Source: CAD feature listing. Evaluate the final solid. Frame: model axes, mm. Coordinates: 2 decimals unless noted, no trailing zeros. One line per question, with ' | ' between items. Start each with the question number.
```python
from build123d import *

# Parameters (mm, degrees)
SKETCH1_W           = 183.7944
SKETCH1_H           = 285.3944
BOSS_EXTRUDE1_DEPTH = 2.9972
SKETCH2_R           = 1.5
BOSS_EXTRUDE2_DEPTH = 2.9972


with BuildPart() as part:
    # Sketch1 → Boss-Extrude1 (new body)
    with BuildSketch(Plane(origin=(0, 0, 0), x_dir=(1, 0, 0), z_dir=(0, 1, 0))):
        Rectangle(SKETCH1_W, SKETCH1_H)
    extrude(amount=BOSS_EXTRUDE1_DEPTH)

    # Sketch2 → Boss-Extrude2 (add)
    # profile 1 of 2: a face of its own
    with BuildSketch(Plane(origin=(0, 2.9972, 0), x_dir=(1, 0, 0), z_dir=(0, 1, 0))):
        with BuildLine():
            Line((-0.300873728, -142.6972), (-91.8972, -142.6972))
            Line((-91.8972, -142.6972), (-91.8972, -180.7972))
            Line((-91.8972, -180.7972), (91.8972, -180.7972))
            Line((91.8972, -180.7972), (91.8972, -142.6972))
            Line((91.8972, -142.6972), (0.300873728, -142.6972))
            ThreePointArc((0.300873728, -142.6972), (0, -160.8022), (-0.300873728, -142.6972))
        make_face()
        with Locations(Location((-14.505, -151.7472, 0), (0, 0, 270))):
            Circle(SKETCH2_R, mode=Mode.SUBTRACT)
        with Locations(Location((14.505, -151.7472, 0), (0, 0, 270))):
            Circle(SKETCH2_R, mode=Mode.SUBTRACT)
    # profile 2 of 2: a face of its own
    with BuildSketch(Plane(origin=(0, 2.9972, 0), x_dir=(1, 0, 0), z_dir=(0, 1, 0))):
        with BuildLine():
            Line((0.300873728, 142.6972), (91.8972, 142.6972))
            Line((91.8972, 142.6972), (91.8972, 180.7972))
            Line((91.8972, 180.7972), (-91.8972, 180.7972))
            Line((-91.8972, 180.7972), (-91.8972, 142.6972))
            Line((-91.8972, 142.6972), (-0.300873728, 142.6972))
            ThreePointArc((-0.300873728, 142.6972), (0, 160.8022), (0.300873728, 142.6972))
        make_face()
        with Locations(Location((-14.505, 151.7472, 0), (0, 0, 270))):
            Circle(SKETCH2_R, mode=Mode.SUBTRACT)
        with Locations(Location((14.505, 151.7472, 0), (0, 0, 270))):
            Circle(SKETCH2_R, mode=Mode.SUBTRACT)
    extrude(amount=-BOSS_EXTRUDE2_DEPTH)


solid = part.part
```
(1) Draft query along Z for faces 1 (the flat face through (-1, 2.997, -3)), 2 (the cylindrical face through (-0.394, 1.52, -160.794)). Return one class per face: pulls with the +Z half, pulls with the -Z half, needs draft (parallel to the pull), parting line crosses it, or undercut.
(2) Contact query for a flat-ended pin moving along its axis: pin 1 Ø2.5 at (x, z) = (-14.5, -151.75) entering from +Y. Output: stop coordinate, or through.
(3) Ray query, L1, parallel to Z at x = 5, y = 0.7; L2, parallel to Z at x = 7, y = 0.5; L3, parallel to X at y = 1.7, z = -154.5. Return the intervals inside material, ascending.
Here are the results:
1) face 1: needs draft | face 2: undercut
2) pin 1: passes through
3) L1: z = -180.8 to -159.3, -144.2 to 144.2, 159.3 to 180.8 | L2: z = -180.8 to -157.49, -146 to 146, 157.49 to 180.8 | L3: x = -91.9 to -8.63, 8.63 to 91.9
